Print and shaded views of the part. All mm, measured from the part's lowest x, y and z. A direction names the side the tool comes from. Round coordinates to 2 decimals unless told otherwise and drop trailing zeros. Write each loop counter-clockwise with the first axis right and the second up, starting at its lowest first coordinate (ties: lowest second). Pieces come first, ordered by that corner, then holes. Notation, with made-up numbers: (19.25, -6.75) - (32.25, -6.75) arc R22 cw to (32.25, 23.25) - close; hole circle Ø9 at (89, -17.5). An arc over 180 degrees is marked (long way). Answer as a JSON object with one key per item and string values. Group by question number.
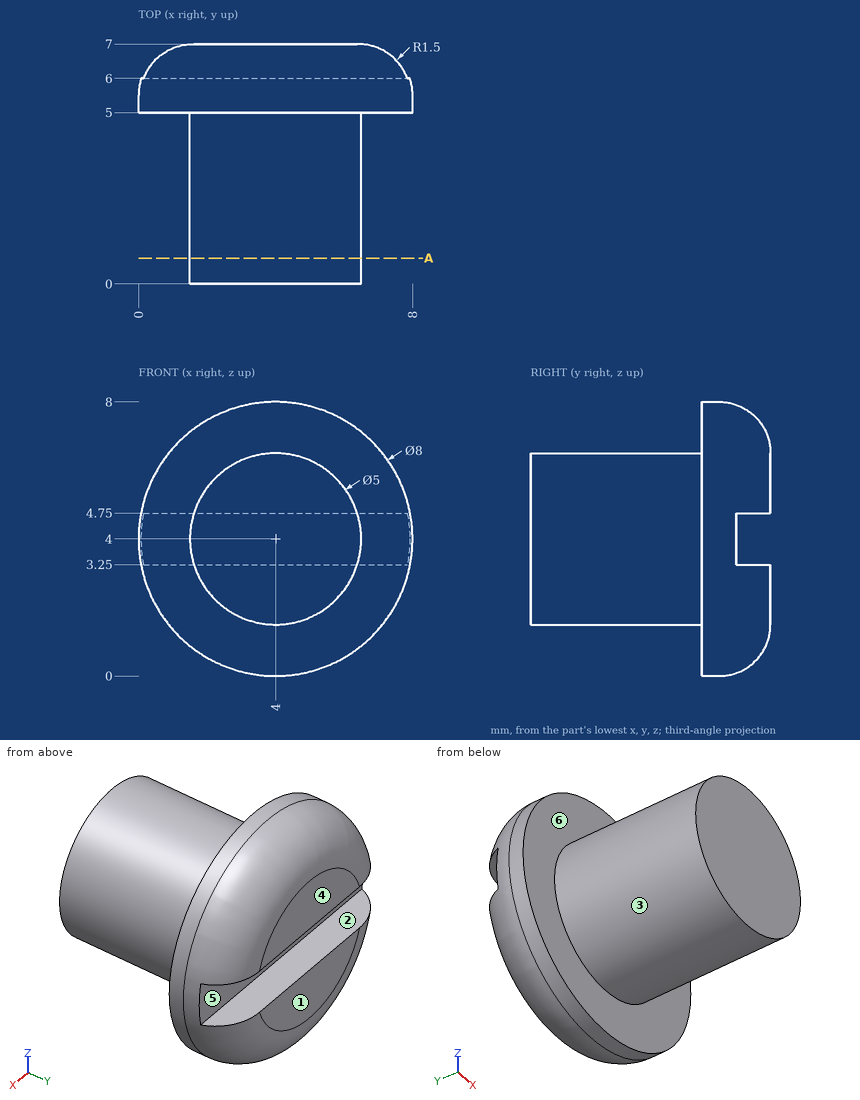
(1) Flat gauge pins, fed straight in: pin 1 (2 mm diameter, centred on x = 1.5, y = 2, fed in from +Z); pin 2 (2 mm diameter, centred on x = 4, z = 6.5, fed in from -Y); pin 3 (0.8 mm diameter, centred on x = 2.5, z = 4, fed in from +Y); pin 4 (1 mm diameter, centred on y = 5.5, z = 5.5, fed in from -X). Where does each tip first touch, or does it go through?
(2) Drill centre lines: line 1 (Z direction, x = 2, y = 6.25); line 2 (Y direction, x = 5.5, z = 4.5); line 3 (Z direction, x = 1.75, y = 6.5). Where is each one in solid material? Low to high. Write a range as from..to.
(3) Pull direction Z, two halves, no side cores. Call the marked faces 1, 2 and 3: pulls with the +Z half, pulls with the -Z half, needs draft (parallel to the pull), parting line crosses it, or undercut.
(4) 3-axis set-ups, long thin cutter, end or side, ignore diameter. For the marked faces 4, 5 and 6: which of +Z, -Z, +X, -X, +Y, -Y reach the whole face in a straight line?
(5) Slice it at A-A (y = 0.75). Write the cut outline in (x, z).
Answer:
{
 "1": {"pin 1": "z = 6", "pin 2": "y = 0", "pin 3": "y = 6", "pin 4": "x = 0.13"},
 "2": {"line 1": "0.77..3.25, 4.75..7.23", "line 2": "0..6", "line 3": "1.17..3.25, 4.75..6.83"},
 "3": {"face 1": "needs draft", "face 2": "undercut", "face 3": "parting line crosses it"},
 "4": {"face 4": "+Z, -Z, +X, -X, +Y", "face 5": "+X, -X, +Y", "face 6": "-Y"},
 "5": {"outline": "circle Ø5 at (4, 4)"}
}
